```python
from build123d import *

# Parameters (mm, degrees)
F1_DEPTH = 25.4
F3_DEPTH = 50.801
F5_DEPTH = 12.701
F7_DEPTH = 12.701


with BuildPart() as f1:
    # F0 (on Front) → F1 (new body)
    with BuildSketch(Plane.XZ):
        Polygon((0, 12.7), (0, 0), (76.2, 0), (76.2, 12.7), (50.8, 12.7), (50.8, 44.45), (25.4, 44.45), (25.4, 12.7), align=None)
    extrude(amount=F1_DEPTH)

    # F2 (on face) → F3 (cut, through all)
    with BuildSketch(Plane.YZ.offset(50.8)):
        with BuildLine():
            ThreePointArc((-19.05, 31.75), (-12.7, 25.4), (-6.35, 31.75))
            Line((-6.35, 31.75), (-19.05, 31.75))
        make_face()
        with BuildLine():
            Line((-19.05, 31.75), (-6.35, 31.75))
            ThreePointArc((-6.35, 31.75), (-12.7, 38.1), (-19.05, 31.75))
        make_face()
        with BuildLine():
            ThreePointArc((-25.4, 31.75), (-12.7, 44.4189396796), (0, 31.75))
            Line((0, 31.75), (0, 44.45))
            Line((0, 44.45), (-25.4, 44.45))
            Line((-25.4, 44.45), (-25.4, 31.75))
        make_face()
    extrude(amount=-F3_DEPTH, mode=Mode.SUBTRACT)

    # F4 (on face) → F5 (cut, through all)
    with BuildSketch(Plane.XY.offset(12.7)):
        with BuildLine():
            ThreePointArc((69.85, -12.7), (67.9901280605, -8.2098719395), (63.5, -6.35))
            Line((63.5, -6.35), (63.5, -19.05))
            ThreePointArc((63.5, -19.05), (67.9901280605, -17.1901280605), (69.85, -12.7))
        make_face()
        with BuildLine():
            Line((63.5, -19.05), (63.5, -6.35))
            ThreePointArc((63.5, -6.35), (57.15, -12.7), (63.5, -19.05))
        make_face()
        with BuildLine():
            Line((76.2, 0), (63.5, 0))
            ThreePointArc((63.5, 0), (76.1671814636, -12.7), (63.5, -25.4))
            Line((63.5, -25.4), (76.2, -25.4))
            Line((76.2, -25.4), (76.2, 0))
        make_face()
    extrude(amount=-F5_DEPTH, mode=Mode.SUBTRACT)

    # F6 (on face) → F7 (cut, through all)
    with BuildSketch(Plane.XY.offset(12.7)):
        with BuildLine():
            ThreePointArc((19.05, -12.7), (17.1901280605, -8.2098719395), (12.7, -6.35))
            Line((12.7, -6.35), (12.7, -19.05))
            ThreePointArc((12.7, -19.05), (17.1901280605, -17.1901280605), (19.05, -12.7))
        make_face()
        with BuildLine():
            Line((12.7, -19.05), (12.7, -6.35))
            ThreePointArc((12.7, -6.35), (6.35, -12.7), (12.7, -19.05))
        make_face()
        with BuildLine():
            ThreePointArc((12.7, -25.4), (0.5314257949, -12.7), (12.7, 0))
            Line((12.7, 0), (0, 0))
            Line((0, 0), (0, -25.4))
            Line((0, -25.4), (12.7, -25.4))
        make_face()
    extrude(amount=-F7_DEPTH, mode=Mode.SUBTRACT)


solid = f1.part
```
Geometry check sheet. Reference: the model listing, model coordinates, mm. A direction names the side the tool comes from. Round coordinates to 2 decimals unless told otherwise and drop trailing zeros. Order: outer loops, then holes, each group sorted by start corner. A loop starts at its lowest first (then second) coordinate and runs counter-clockwise, first axis right, second up. Notation, with made-up numbers: (86.25, 35.25) - (135.25, 35.25) arc R32 cw to (135.25, 71.25) - close; hole circle Ø11 at (73.5, 35). An arc over 180 degrees is marked (long way). Use a Markdown table: item, result. Add a question column.
1) Gauge pin test, flat ends, axial feed: P1, Ø2, axis at x = 9.5, y = -20.5, coming from the +Z side; P2, Ø12, axis at y = -6, z = 7, coming from the +X side; P3, Ø3, axis at y = -9.5, z = 6.5, coming from the -X side. Record the tip position at first contact, or that the pin passes through.
2) Section check D-D (z = 21). Record the cut outline in (x, y), then the cut area to 3 significant figures.
3) Thickness scan on line 1 along Z through (x, y) = (40.5, -12.7); line 2 along X through (y, z) = (-13.5, 6); line 3 along X through (y, z) = (-7.25, 11.5). Record the ranges inside material, lowest first.
4) Section check C-C (y = -3). Record the cut outline in (x, z).
5) Section check B-B (y = -16.75). Record the cut outline in (x, z), then the cut area to 3 significant figures.
6) Set-up check for faces 5 (the flat face through (50.8, -13, 25)), 6 (the cylindrical face through (38.278, -12.979, 44.416)), 7 (the flat face through (19, -15, 12.7)): record each of +Z, -Z, +X, -X, +Y, -Y from which the full face is reachable in a straight line by a thin tool's end or side.
7) Section check A-A (x = 60). Record the cut outline in (y, z).
8) Mould release check, pull along Y, two halves, no side actions. Record for faces 1 (the flat face through (38, -25.4, 13)), 2 (the flat face through (55, -13, 12.7)), 3 (the cylindrical face through (38.3, -9.8, 26.1)), 4 (the cylindrical face through (0.534, -12.972, 6.439)): released by +Y, released by -Y, zero draft, split by the parting line, or undercut.
Established:
| question | item | result |
|---|---|---|
| 1 | P1 | z = 12.7 |
| 1 | P2 | x = 76.15 |
| 1 | P3 | x = 0.65 |
| 2 | outline | (25.4, -25.4) - (50.8, -25.4) - (50.8, 0) - (25.4, 0) - close |
| 2 | area | 645 mm2 |
| 3 | line 1 | 0 to 25.4, 38.1 to 44.42 |
| 3 | line 2 | 0.56 to 6.4, 19 to 57.2, 69.8 to 76.14 |
| 3 | line 3 | 1.76 to 9.44, 15.96 to 60.24, 66.76 to 74.94 |
| 4 | outline | (5.03, 0) - (71.66, 0) - (71.66, 12.7) - (50.8, 12.7) - (50.8, 39.92) - (25.4, 39.92) - (25.4, 12.7) - (5.03, 12.7) - close |
| 5 | outline | (1.19, 0) - (7.81, 0) - (7.81, 12.7) - (1.19, 12.7) - close; (17.59, 0) - (58.61, 0) - (58.61, 12.7) - (50.8, 12.7) - (50.8, 26.86) - (25.4, 26.86) - (25.4, 12.7) - (17.59, 12.7) - close; (25.4, 36.64) - (50.8, 36.64) - (50.8, 43.76) - (25.4, 43.76) - close; (68.39, 0) - (75.5, 0) - (75.5, 12.7) - (68.39, 12.7) - close |
| 5 | area | 1,240 mm2 |
| 6 | face 5 | +Z, +X, +Y, -Y |
| 6 | face 6 | +Z, +X, -X |
| 6 | face 7 | +Z, -X, +Y, -Y |
| 7 | outline | (-25.4, 0) - (-18, 0) - (-18, 12.7) - (-25.4, 12.7) - close; (-7.4, 0) - (0, 0) - (0, 12.7) - (-7.4, 12.7) - close |
| 8 | face 1 | released by -Y |
| 8 | face 2 | zero draft |
| 8 | face 3 | undercut |
| 8 | face 4 | split by the parting line |
